Could you check a few things on this model? Use its own coordinates, in mm. Face numbers are marked on the shaded views. A direction names the side the tool comes from. Give positions to 0.01 mm unless a question says otherwise; leave off trailing zeros. Order: outer loops, then holes, each group sorted by start corner. A loop starts at its lowest first (then second) coordinate and runs counter-clockwise, first axis right, second up. Notation, with made-up numbers: M 42.25,21.25 L 51.25,21.25 A19 ccw 51.25,30.25 Z; hole C 79.5,10 d3. An arc over 180 degrees is marked long. Use a Markdown table: item, result. Add a question column.
Item 1: I'm going to push flat-ended pins straight in: pin 1 Ø2.5 at (y, z) = (16, 4.5) entering from +X; pin 2 Ø1.5 at (x, z) = (-28.5, -1.5) entering from +Y; pin 3 Ø3.5 at (y, z) = (7, 0.5) entering from -X. Where does each tip first touch, or does it pass through?
Item 2: Suppose I cut it at C-C on y = 7. Write out the boundary of the cut face in (x, z).
Item 3: Suppose I cut it at A-A on x = 0. Write out the boundary of the cut face in (y, z), plus the area to 3 significant figures.
Item 4: For the marked faces 1, 2 and 3, which set-ups out of +Z, -Z, +X, -X, +Y, -Y let a thin tool reach every point of the face, with its end or its side?
Item 5: Suppose I cut it at D-D on x = -32.5. Write out the boundary of the cut face in (y, z).
Item 6: If I drill on L1, parallel to Y at x = -17, z = 1; L2, parallel to Y at x = 6, z = -5.75; L3, parallel to Z at x = -34.5, y = 3.25, over which ranges is the centre line in solid material (lowest first)? Write a range as from..to.
Item 7: If we mould it in two halves opening along X, with no side actions, what happens to the marked faces 4, 5 and 6? For each: released by +X, released by -X, zero draft, split by the parting line, or undercut.
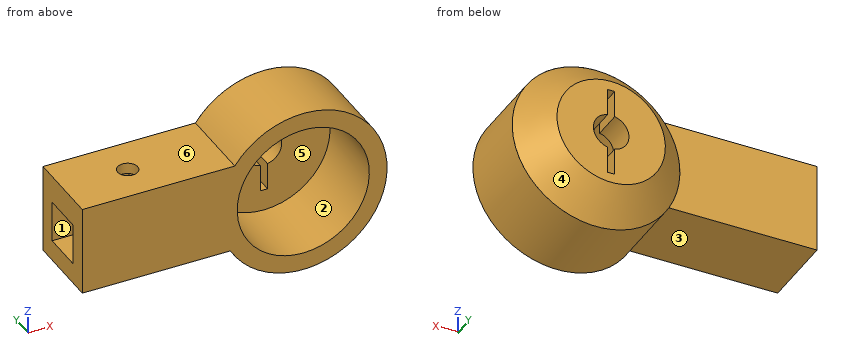
from build123d import *

# Parameters (mm, degrees)
ESBO_O2_R                = 11.15
RESSALTO_EXTRUS_O1_DEPTH = 13
ESBO_O3_W                = 7
ESBO_O3_H                = 7
CORTE_EXTRUS_O1_DEPTH    = 26
CORTE_EXTRUS_O2_DEPTH    = 2.8
ESBO_O10_R               = 1.683661958
CORTE_EXTRUS_O3_DEPTH    = 2.8
ESBO_O11_R               = 14.15
RESSALTO_EXTRUS_O2_DEPTH = 5
CHANFRO1_SIZE            = 5


with BuildPart() as part:
    # Esboço2 → Ressalto-extrusão1 (new body)
    with BuildSketch(Plane(origin=(0, 0, 0), x_dir=(1, 0, 0), z_dir=(0, 1, 0))):
        with BuildLine():
            Line((-12.297255791, 7), (-37.297255791, 7))
            Line((-37.297255791, 7), (-37.297255791, -8.161034979))
            Line((-37.297255791, -8.161034979), (-11.559412099, -8.161034979))
            ThreePointArc((-11.559412099, -8.161034979), (14.133272661, 0.687825475), (-12.297255791, 7))
        make_face()
        with Locations(Location((0, 0, 0), (0, 0, 90))):
            Circle(ESBO_O2_R, mode=Mode.SUBTRACT)
    extrude(amount=RESSALTO_EXTRUS_O1_DEPTH)

    # Esboço3 → Corte-extrusão1 (cut)
    with BuildSketch(Plane.ZY.offset(37.297255791)):
        with Locations((0, 6.5)):
            Rectangle(ESBO_O3_W, ESBO_O3_H)
    extrude(amount=-CORTE_EXTRUS_O1_DEPTH, mode=Mode.SUBTRACT)

    # Esboço7 → Corte-extrusão2 (cut)
    with BuildSketch(Plane(origin=(0, 0, 3.5), x_dir=(-1, 0, 0), z_dir=(0, 0, -1))):
        Polygon((22.62619922, 6.5), (24.473720081, 3.3), (28.168761804, 3.3), (30.016282665, 6.5), (28.168761804, 9.7), (24.473720081, 9.7), align=None)
    extrude(amount=-CORTE_EXTRUS_O2_DEPTH, mode=Mode.SUBTRACT)

    # Esboço10 → Corte-extrusão3 (cut)
    with BuildSketch(Plane(origin=(0, 0, 6.3), x_dir=(-1, 0, 0), z_dir=(0, 0, -1))):
        with Locations((26.321240942, 6.5)):
            Circle(ESBO_O10_R)
    extrude(amount=-CORTE_EXTRUS_O3_DEPTH, mode=Mode.SUBTRACT)

    # Esboço11 → Ressalto-extrusão2 (add)
    with BuildSketch(Plane(origin=(0, 13, 0), x_dir=(1, 0, 0), z_dir=(0, 1, 0))):
        with Locations(Location((0, 0, 0), (0, 0, 150.350053351))):
            Circle(ESBO_O11_R)
        with BuildLine():
            Line((0.6, -7.5), (0.6, -2.939387691))
            ThreePointArc((0.6, -2.939387691), (3, 0), (0.6, 2.939387691))
            Line((0.6, 2.939387691), (0.6, 7.5))
            Line((0.6, 7.5), (-0.6, 7.5))
            Line((-0.6, 7.5), (-0.6, 2.939387691))
            ThreePointArc((-0.6, 2.939387691), (-3, 0), (-0.6, -2.939387691))
            Line((-0.6, -2.939387691), (-0.6, -7.5))
            Line((-0.6, -7.5), (0.6, -7.5))
        make_face(mode=Mode.SUBTRACT)
    extrude(amount=RESSALTO_EXTRUS_O2_DEPTH)

    # Chanfro1
    chanfro1_edges = [part.edges().sort_by_distance(p)[0] for p in [
        (12.297255791, 18, 7),
    ]]
    chamfer(chanfro1_edges, length=CHANFRO1_SIZE - 0.0001)  # a hair under: the kernel refuses the full size


solid = part.part
Findings below:
| question | item | result |
|---|---|---|
| 1 | pin 1 | stops at x = 11.63 |
| 1 | pin 2 | stops at y = 13 |
| 1 | pin 3 | stops at x = -11.3 |
| 2 | outline | M -37.3,-7 L -12.3,-7 A14.15 ccw long -11.56,8.16 L -24.71,8.16 L -24.71,6.3 L -22.91,6.3 L -22.91,3.5 L -11.3,3.5 L -11.3,-3.5 L -37.3,-3.5 Z; M -37.3,3.5 L -29.73,3.5 L -29.73,6.3 L -27.93,6.3 L -27.93,8.16 L -37.3,8.16 Z; hole C 0,0 d22.3 |
| 3 | outline | M 0,-14.15 L 13,-14.15 L 18,-9.15 L 18,-7.5 L 13,-7.5 L 13,-11.15 L 0,-11.15 Z; M 0,11.15 L 13,11.15 L 13,7.5 L 18,7.5 L 18,9.15 L 13,14.15 L 0,14.15 Z |
| 3 | area | 120 mm^2 |
| 4 | face 1 | -X |
| 4 | face 2 | -Y |
| 4 | face 3 | -Z, -X, +Y, -Y |
| 5 | outline | M 0,-7 L 13,-7 L 13,8.16 L 0,8.16 Z; hole M 3,-3.5 L 10,-3.5 L 10,3.5 L 3,3.5 Z |
| 6 | L1 | y = 0..3, 10..13 |
| 6 | L2 | y = 13..18 |
| 6 | L3 | z = -7..-3.5, 3.5..8.16 |
| 7 | face 4 | split by the parting line |
| 7 | face 5 | undercut |
| 7 | face 6 | zero draft |
